```python
from build123d import *

# Parameters (mm, degrees)
F0_W     = 6
F0_H     = 6
F0_R     = 1.75
F2_DEPTH = 18
F1_W     = 9.8
F1_H     = 18
F3_DEPTH = 3
F4_W     = 10
F4_H     = 10
F5_DEPTH = 20
F8_DEPTH = 25
F9_DEPTH = 25


with BuildPart() as f2:
    # F0 (on Top) → F2 (new body)
    with BuildSketch(Plane.XY):
        Polygon((12.5, 9), (-12.5, 9), (-12.5, 3), (-12.5, -9), (12.5, -9), (12.5, 3), align=None)
        with BuildLine():
            ThreePointArc((-13.75, 6), (-16.737437, 7.237437), (-15.5, 4.25))
            ThreePointArc((-15.5, 4.25), (-14.262563, 4.762563), (-13.75, 6))
        make_face()
        Polygon((-12.5, 3), (-12.5, 9), (-18.5, 9), (-18.5, 3), (-15.5, 3), align=None)
        with BuildLine():
            ThreePointArc((-13.75, 6), (-14.262563, 4.762563), (-15.5, 4.25))
            ThreePointArc((-15.5, 4.25), (-16.737437, 7.237437), (-13.75, 6))
        make_face(mode=Mode.SUBTRACT)
        with Locations((15.5, 6)):
            Rectangle(F0_W, F0_H)
        with Locations((15.5, 6)):
            Circle(F0_R, mode=Mode.SUBTRACT)
    extrude(amount=F2_DEPTH)

    # F1 (on face) → F3 (cut)
    with BuildSketch(Plane.XY):
        Rectangle(F1_W, F1_H)
    extrude(amount=F3_DEPTH, mode=Mode.SUBTRACT)

    # F4 (on face) → F5 (cut)
    with BuildSketch(Plane.XZ.offset(9)):
        with Locations((5, 10)):
            Rectangle(F4_W, F4_H)
        with Locations((-5, 10)):
            Rectangle(F4_W, F4_H)
    extrude(amount=-F5_DEPTH, mode=Mode.SUBTRACT)

    # F7 (on face) → F8 (cut)
    with BuildSketch(Plane(origin=(-12.5, 0, 0), x_dir=(0, -1, 0), z_dir=(-1, 0, 0))):
        Polygon((0.850376, 18), (9, 6.250017), (9, 18), align=None)
    extrude(amount=-F8_DEPTH, mode=Mode.SUBTRACT)

    # F6 (on face) → F9 (cut)
    with BuildSketch(Plane.XY.offset(18)):
        with BuildLine():
            ThreePointArc((2, 3.8), (-1.414214, 5.214214), (0, 1.8))
            ThreePointArc((0, 1.8), (1.414214, 2.385786), (2, 3.8))
        make_face()
        with BuildLine():
            ThreePointArc((0, -4.25), (-1.75, -6), (0, -7.75))
            Line((0, -7.75), (0, -6))
            Line((0, -6), (0, -4.25))
        make_face()
        with BuildLine():
            Line((0, -6), (0, -7.75))
            ThreePointArc((0, -7.75), (1.237437, -7.237437), (1.75, -6))
            ThreePointArc((1.75, -6), (1.237437, -4.762563), (0, -4.25))
            Line((0, -4.25), (0, -6))
        make_face()
    extrude(amount=-F9_DEPTH, mode=Mode.SUBTRACT)


solid = f2.part
```
Work out the finished part from the listing and answer in its coordinate system (mm). A direction names the side the tool comes from. Coordinates: 2 decimals unless noted, no trailing zeros. Order: outer loops, then holes, each group sorted by start corner. A loop starts at its lowest first (then second) coordinate and runs counter-clockwise, first axis right, second up. Notation, with made-up numbers: (58, 40.5) - (114, 40.5) arc R28 ccw to (114, 67.5) - close; hole circle Ø7 at (-1.5, 34.25). An arc over 180 degrees is marked (long way). Answer as a JSON object with one key per item and string values.
1. A tool of negligible diameter and unlimited length cuts with its end or side. For faces 4 (the face through (-16, 3, 9)), 5 (the face through (15, 3, 9)), 6 (the face through (-4.9, 0, 1)), 7 (the face through (10, 2, 10)), from which of +Z, -Z, +X, -X, +Y, -Y can it reach the whole face along a straight path? Write none if from no direction.
Output values:
{"face 4": "+Z, -Z, -X, -Y", "face 5": "+Z, -Z, +X, -Y", "face 6": "-Z, +Y, -Y", "face 7": "+Y, -Y"}
2. Find section A-A on z = 10.5. Determine the outline of the cut face in (x, y).
Output values:
{"outline": "(-18.5, 3) - (-12.5, 3) - (-12.5, -6.05) - (-10, -6.05) - (-10, 9) - (-18.5, 9) - close; (10, -6.05) - (12.5, -6.05) - (12.5, 3) - (18.5, 3) - (18.5, 9) - (10, 9) - close; hole circle Ø3.5 at (-15.5, 6); hole circle Ø3.5 at (15.5, 6)"}
3. Find section D-D on y = 6.75. Determine the outline of the cut face in (x, z), plus the area to 3 significant figures.
Output values:
{"outline": "(-18.5, 0) - (-17.08, 0) - (-17.08, 18) - (-18.5, 18) - close; (-13.92, 0) - (-4.9, 0) - (-4.9, 3) - (4.9, 3) - (4.9, 0) - (13.92, 0) - (13.92, 18) - (-13.92, 18) - close; (17.08, 0) - (18.5, 0) - (18.5, 18) - (17.08, 18) - close; hole (-10, 5) - (10, 5) - (10, 15) - (-10, 15) - close", "area": "323 mm²"}
4. Find section C-C on y = 0.75. Determine the outline of the cut face in (x, z).
Output values:
{"outline": "(-12.5, 0) - (-4.9, 0) - (-4.9, 3) - (4.9, 3) - (4.9, 0) - (12.5, 0) - (12.5, 18) - (-12.5, 18) - close; hole (-10, 5) - (10, 5) - (10, 15) - (-10, 15) - close"}
5. The mould has two halves that part along X. Classify faces 1 (the face through (12.5, -2, 7)), 2 (the face through (0, -9, 4)), 3 (the face through (0, 0, 3)): +X half, -X half, draft (parallel to the pull), parting line (faces both ways), or undercut.
Output values:
{"face 1": "+X half", "face 2": "draft", "face 3": "undercut"}
6. Each of these flat-tipped pins is pushed along its axis until it touches: P1, Ø3, axis at y = 1, z = 11.5, coming from the +X side; P2, Ø3, axis at x = -16, z = 7.5, coming from the -Y side; P3, Ø2, axis at x = 6, y = 6.5, coming from the -Z side; P4, Ø10, axis at y = -6.5, z = 9.5, coming from the -X side. Where does it stop, or does it pass through?
Output values:
{"P1": "stops at x = 12.5", "P2": "stops at y = 3", "P3": "stops at z = 0", "P4": "stops at x = -12.5"}
7. Consider line 1 (X direction, y = 3.8, z = 3.75); line 2 (X direction, y = 6.5, z = 11.75); line 3 (Z direction, x = 7, y = 6.25). Determine where each line is inside the solid, lowest interval first.
Output values:
{"line 1": "x = -18.5 to -2, 2 to 18.5", "line 2": "x = -18.5 to -17.18, -13.82 to -10, 10 to 13.82, 17.18 to 18.5", "line 3": "z = 0 to 5, 15 to 18"}
8. Find section B-B on x = -3. Determine the outline of the cut face in (y, z), plus the area to 3 significant figures.
Output values:
{"outline": "(-9, 3) - (9, 3) - (9, 5) - (-9, 5) - close; (-2.93, 15) - (9, 15) - (9, 18) - (-0.85, 18) - close", "area": "68.7 mm²"}
